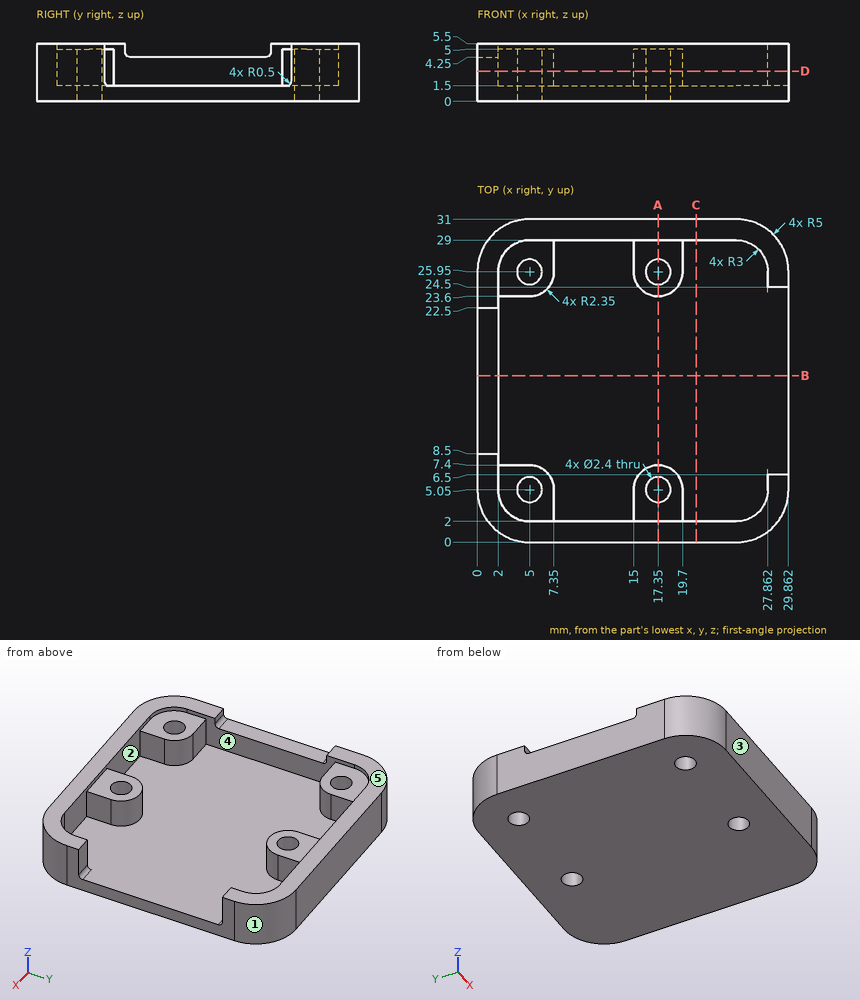
Drawing for the job (mm, zero at the part's lowest x, y, z). A direction names the side the tool comes from. Give positions to 0.01 mm unless a question says otherwise; leave off trailing zeros. Loops run counter-clockwise (first coordinate to the right, second up) from the corner with the lowest first, then second, coordinate; pieces in that order, holes last.
(1) Band-saw the part on B-B (y = 16). Write the cut outline in (x, z).
Return value:
outline: (0, 0) - (29.86, 0) - (29.86, 1.5) - (2, 1.5) - (2, 4.25) - (0, 4.25) - close
(2) Band-saw the part on C-C (x = 21). Write the cut outline in (y, z).
Return value:
outline: (0, 0) - (31, 0) - (31, 5.5) - (29, 5.5) - (29, 1.5) - (2, 1.5) - (2, 5.5) - (0, 5.5) - close
(3) Drill centre lines: line 1 along X through (y, z) = (4, 2.6); line 2 along Y through (x, z) = (17.35, 1.55); line 3 along X through (y, z) = (27.5, 3.4). Where is each one in solid material? Low to high.
Return value:
line 1: x = 0.1 to 4.42, 5.58 to 7.35, 15 to 16.77, 17.93 to 19.7, 27.69 to 29.76
line 2: y = 0 to 3.85, 6.25 to 7.4, 23.6 to 24.75, 27.15 to 31
line 3: x = 0.23 to 7.35, 15 to 19.7, 27.46 to 29.63
(4) Pull direction Y, two halves, no side cores. Call the marked faces 3, 4 and 5: pulls with the +Y half, pulls with the -Y half, needs draft (parallel to the pull), parting line crosses it, or undercut.
Return value:
face 3: pulls with the -Y half
face 4: undercut
face 5: needs draft
(5) Band-saw the part on D-D (z = 2.9). Count the separate pieces of the cut face and the enclosed holes in it, and give its area (3 significant figures).
Return value:
separate pieces: 1
enclosed holes: 4
area: 257 mm2
(6) Band-saw the part on A-A (x = 17.35). Write the cut outline in (y, z), and give its area (3 significant figures).
Return value:
outline: (0, 0) - (3.85, 0) - (3.85, 5) - (2, 5) - (2, 5.5) - (0, 5.5) - close; (6.25, 0) - (24.75, 0) - (24.75, 5) - (23.6, 5) - (23.6, 1.5) - (7.4, 1.5) - (7.4, 5) - (6.25, 5) - close; (27.15, 0) - (31, 0) - (31, 5.5) - (29, 5.5) - (29, 5) - (27.15, 5) - close
area: 76.3 mm2
(7) 3-axis set-ups, long thin cutter, end or side, ignore diameter. For the marked faces 1 and 2: which of +Z, -Z, +X, -X, +Y, -Y reach the whole face in a straight line?
Return value:
face 1: +Z, -Z, +X, +Y
face 2: +Z
(8) Pin check, flat tips, straight feed: pin 1 (3 mm diameter, centred on x = 25, y = 23, fed in from -Z); pin 2 (4 mm diameter, centred on x = 5, y = 5.05, fed in from +Z); pin 3 (8 mm diameter, centred on x = 10.5, y = 19.5, fed in from +Z); pin 4 (0.9 mm diameter, centred on y = 3, z = 3.5, fed in from -X). Stop position of each tip, or through.
Return value:
pin 1: stops at z = 0
pin 2: stops at z = 5
pin 3: stops at z = 1.5
pin 4: stops at x = 0.25
